Here's how the part is built. I have some questions about the finished solid (model axes, mm). A direction names the side the tool comes from. Coordinates: 2 decimals unless noted, no trailing zeros. Write each loop counter-clockwise with the first axis right and the second up, starting at its lowest first coordinate (ties: lowest second). Pieces come first, ordered by that corner, then holes. Notation, with made-up numbers: M 50.25,23 L 72.25,23 A18 ccw 72.25,57 Z; hole C -15.75,-12.75 d4. An arc over 180 degrees is marked long. Use a Markdown table: item, result.
```python
from build123d import *

# Parameters (mm, degrees)
SKETCH_W        = 25
SKETCH_H        = 20
SKETCH_R        = 3.85
PAD_DEPTH       = 11
PAD001_DEPTH    = 25
POCKET_DEPTH    = 7.06
SKETCH003_R     = 1.6
POCKET001_DEPTH = 12.561
FILLET_R        = 3
FILLET001_R     = 1


with BuildPart() as part:
    # Sketch → Pad (new body)
    with BuildSketch(Plane.XY):
        Rectangle(SKETCH_W, SKETCH_H)
        Circle(SKETCH_R, mode=Mode.SUBTRACT)
    extrude(amount=PAD_DEPTH)

    # Sketch001 (on Face4 of Pad) → Pad001 (join)
    with BuildSketch(Plane(origin=(-12.5, 0, 0), x_dir=(0, -1, 0), z_dir=(-1, 0, 0))):
        Polygon((0, 0), (-4.74, 0), (-2.94, -1.56), (2.94, -1.56), (4.74, 0), align=None)
    extrude(amount=-PAD001_DEPTH)

    # Sketch002 (on Face13 of Pad001) → Pocket (cut)
    with BuildSketch(Plane(origin=(0, 0, -1.56), x_dir=(1, 0, 0), z_dir=(0, 0, -1))):
        Polygon((0, -7.188011), (6.225, -3.594005), (6.225, 3.594005), (0, 7.188011), (-6.225, 3.594005), (-6.225, -3.594005), align=None)
    extrude(amount=-POCKET_DEPTH, mode=Mode.SUBTRACT)

    # Sketch003 (on Face19 of Pocket) → Pocket001 (cut, through all)
    with BuildSketch(Plane(origin=(0, 0, -1.56), x_dir=(1, 0, 0), z_dir=(0, 0, -1))):
        with Locations((-9.3625, 0)):
            Circle(SKETCH003_R)
        with Locations((9.3625, 0)):
            Circle(SKETCH003_R)
    extrude(amount=-POCKET001_DEPTH, mode=Mode.SUBTRACT)

    # Fillet
    fillet_edges = [part.edges().sort_by_distance(p)[0] for p in [
        (12.5, -10, 5.5),
        (12.5, 10, 5.5),
        (-12.5, 10, 5.5),
        (-12.5, -10, 5.5),
    ]]
    fillet(fillet_edges, radius=FILLET_R)

    # Fillet001
    fillet001_edges = [part.edges().sort_by_distance(p)[0] for p in [
        (-3.85, 0, 5.5),
    ]]
    fillet(fillet001_edges, radius=FILLET001_R)


solid = part.part
```
1. Suppose I cut it at A-A on y = 0. State how many separate pieces and enclosed holes the cut face has, and give its area (3 significant figures).
Answers follow:
| item | result |
|---|---|
| separate pieces | 4 |
| enclosed holes | 0 |
| area | 103 mm2 |
2. Suppose I cut it at C-C on x = -8.5. Write out the boundary of the cut face in (y, z).
Answers follow:
| item | result |
|---|---|
| outline | M -10,0 L -4.74,0 L -2.94,-1.56 L -1.35,-1.56 L -1.35,11 L -10,11 Z; M 1.35,-1.56 L 2.94,-1.56 L 4.74,0 L 10,0 L 10,11 L 1.35,11 Z |
3. I need wall thicknesses on probe 1 along X at (y, z) = (0, 8.5); probe 2 along X at (y, z) = (0, 1.5) (1 decimal); probe 3 along Y at (x, z) = (-9.5, 8.25). Which ranges of each line are inside material? Lowest first, please.
Answers follow:
| item | result |
|---|---|
| probe 1 | x = -12.5 to -10.96, -7.76 to -3.85, 3.85 to 7.76, 10.96 to 12.5 |
| probe 2 | x = -12.5 to -11, -7.8 to -6.2, 6.2 to 7.8, 11 to 12.5 |
| probe 3 | y = -10 to -1.59, 1.59 to 10 |
4. Will these pins go through, and if not, where does the flat tip stop? pin 1 Ø4 at (x, y) = (2.5, 7.5) entering from -Z; pin 2 Ø1.9 at (x, y) = (9.36, 0) entering from -Z; pin 3 Ø3.5 at (x, y) = (1.5, -2.5) entering from -Z.
Answers follow:
| item | result |
|---|---|
| pin 1 | stops at z = 0 |
| pin 2 | passes through |
| pin 3 | stops at z = 5.52 |
5. We'd pull the mould along Y, two halves only. Please class faces 1 (the face through (0, 5, 11)), 2 (the face through (0, 10, 5)), 3 (the face through (3.1, 5.4, 2.2)), 4 (the face through (-4, 3, 5.5)): +Y half, -Y half, draft (parallel to the pull), parting line (faces both ways), or undercut.
Answers follow:
| item | result |
|---|---|
| face 1 | draft |
| face 2 | +Y half |
| face 3 | undercut |
| face 4 | undercut |
6. Suppose I cut it at D-D on y = 6. Write out the boundary of the cut face in (x, z), and give its area (3 significant figures).
Answers follow:
| item | result |
|---|---|
| outline | M -12.5,0 L -2.06,0 L -2.06,5.5 L 2.06,5.5 L 2.06,0 L 12.5,0 L 12.5,11 L -12.5,11 Z |
| area | 252 mm2 |
7. Which directions (+Z, -Z, +X, -X, +Y, -Y) give clear straight access to the entire face, cutting with the end or side of a thin tool? Please do faces 5 (the face through (-7.836, -0.481, 4.632)), 6 (the face through (-3.156, 5.366, 2.208)), 7 (the face through (-0.2, -7.3, 0)).
Answers follow:
| item | result |
|---|---|
| face 5 | +Z, -Z |
| face 6 | -Z |
| face 7 | -Z, +X, -X, -Y |
8. Suppose I cut it at B-B on z = 0.75. Write out the boundary of the cut face in (x, y) (1 decimal).
Answers follow:
| item | result |
|---|---|
| outline | M -12.5,-7 A3 ccw -9.5,-10 L 9.5,-10 A3 ccw 12.5,-7 L 12.5,7 A3 ccw 9.5,10 L -9.5,10 A3 ccw -12.5,7 Z; hole C -9.4,0 d3.2; hole M -6.2,-3.6 L 0,-7.2 L 6.2,-3.6 L 6.2,3.6 L 0,7.2 L -6.2,3.6 Z; hole C 9.4,0 d3.2 |
